Part model, mm, in its own coordinate system. Give positions to 0.01 mm unless a question says otherwise; leave off trailing zeros. Write each loop counter-clockwise with the first axis right and the second up, starting at its lowest first coordinate (ties: lowest second). Pieces come first, ordered by that corner, then holes. Notation, with made-up numbers: M 23.5,59.25 L 28.5,59.25 A6 cw 28.5,63.25 Z; hole C -5.75,31.25 d11. An arc over 180 degrees is marked long. Use CSV: the item, a comma, the result in double quotes. Start each with the question number.
Item 1: Drill centre lines: line 1 (Y direction, x = 16, z = 0.7); line 2 (Y direction, x = 10, z = 1.2); line 3 (Z direction, x = 26.5, y = 15). Where is each one in solid material? Low to high. Write a range as [from, to].
Item 2: Cut at A-A (x = 12). List the corners of the cut face in (y, z).
Item 3: Cut at B-B (y = 10.75). List the corners of the cut face in (x, z), then the cut area to 3 significant figures.
Item 4: Pin check, flat tips, straight feed: pin 1 (0.6 mm diameter, centred on y = 7, z = 1.5, fed in from +X); pin 2 (0.6 mm diameter, centred on y = 7, z = 1, fed in from -X). Stop position of each tip, or through.
Autodesk Inventor part; units mm, degrees
ref_plane "YZ Plane" through (0, 0, 0) normal (1, 0, 0) x (0, 1, 0)
ref_plane "XZ Plane" through (0, 0, 0) normal (0, 1, 0) x (-1, 0, 0)
ref_plane "XY Plane" through (0, 0, 0) normal (0, 0, 1) x (1, 0, 0)
sketch "Sketch1" plane through (0, 0, 0) normal (0, 0, 1) x (1, 0, 0)
  line L0 (0, 0) -> (0, 16.7)
  line L1 (0, 16.7) -> (34.5, 16.7)
  line L2 (34.5, 16.7) -> (34.5, 0)
  line L3 (34.5, 0) -> (0, 0)
  dimension "d0" = 16.7
  dimension "d1" = 34.5
extrude "Extrusion1" add sketch "Sketch1" along normal blind 1
sketch "Sketch2" plane through (0, 0, 1) normal (0, 0, 1) x (1, 0, 0)
  line L0 (0, 16.7) -> (0, 0)
  line L1 (0, 0) -> (34.5, 0)
  line L2 (0, 9.2) -> (34.5, 9.2)
  line L3 (34.5, 9.2) -> (34.5, 7.5)
  line L4 (34.5, 7.5) -> (0, 7.5)
  line L5 (0, 7.5) -> (0, 9.2)
  dimension "d4" = 34.5
  dimension "d5" = 1.7
  dimension "d6" = 7.5
extrude "Extrusion2" cut sketch "Sketch2" against normal blind 0.5
sketch "Sketch3" plane through (0, 0, 0.5) normal (0, 0, 1) x (1, 0, 0)
  line L0 (34.5, 7.5) -> (0, 7.5)
  line L1 (34.5, 7.5) -> (0, 7.5)
  line L2 (0, 9.2) -> (0.5, 9.2)
  line L3 (0.5, 9.2) -> (0.5, 7.5)
  line L4 (0.5, 7.5) -> (0, 7.5)
  line L5 (0, 7.5) -> (0, 9.2)
  line L6 (34.5, 9.2) -> (34, 9.2)
  line L7 (34, 9.2) -> (34, 7.5)
  line L8 (34, 7.5) -> (34.5, 7.5)
  line L9 (34.5, 7.5) -> (34.5, 9.2)
  point P0 (0, 0)
  dimension "d9" = 0.5
  dimension "d10" = 0.5
extrude "Extrusion3" add sketch "Sketch3" along normal blind 0.5
sketch "Sketch4" plane through (0, 0, 1) normal (0, 0, 1) x (1, 0, 0)
  line L0 (0.5, 10.2) -> (34, 10.2)
  line L1 (34, 10.2) -> (34, 9.2)
  line L2 (34, 9.2) -> (0.5, 9.2)
  line L3 (0.5, 9.2) -> (0.5, 10.2)
  line L4 (34, 7.5) -> (0.5, 7.5)
  line L5 (0.5, 7.5) -> (0.5, 6.5)
  line L6 (0.5, 6.5) -> (34, 6.5)
  line L7 (34, 6.5) -> (34, 7.5)
  dimension "d13" = 1
  dimension "d14" = 1
extrude "Extrusion4" add sketch "Sketch4" along normal blind 0.5
properties part number "Zijplaat 2"
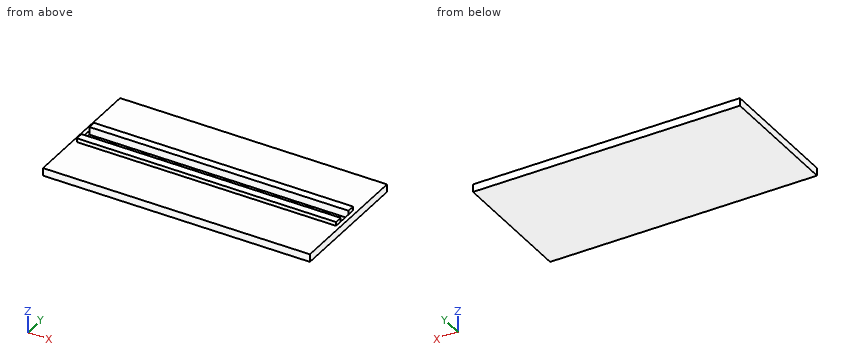
Worked answers:
1,line 1,"y = [0, 7.5], [9.2, 16.7]"
1,line 2,"y = [6.5, 7.5], [9.2, 10.2]"
1,line 3,"z = [0, 1]"
2,outline,"M 0,0 L 16.7,0 L 16.7,1 L 10.2,1 L 10.2,1.5 L 9.2,1.5 L 9.2,0.5 L 7.5,0.5 L 7.5,1.5 L 6.5,1.5 L 6.5,1 L 0,1 Z"
3,outline,"M 0,0 L 34.5,0 L 34.5,1 L 0,1 Z"
3,area,"34.5 mm^2"
4,pin 1,"stops at x = 34"
4,pin 2,"stops at x = 0"
